Input: part model. Units: mm. Frame: model coordinates. Round coordinates to 2 decimals unless told otherwise and drop trailing zeros. Write each loop counter-clockwise with the first axis right and the second up, starting at its lowest first coordinate (ties: lowest second). Pieces come first, ordered by that corner, then holes. Notation, with made-up numbers: (65, 24) -> (78, 24) arc R25 ccw to (78, 57) -> close; hole circle Ø7 at (-12.75, 32). An arc over 180 degrees is marked (long way). Write item = value, one per line. Start each with the question number.
```python
from build123d import *

# Parameters (mm, degrees)
BOSS_EXTRUDE1_DEPTH  = 3.000000492
CUT_EXTRUDE1_DEPTH   = 4.000000492
BOSS_EXTRUDE3_DEPTH  = 4.999998957
SKETCH14_R           = 2.583283714
CUT_EXTRUDE6_DEPTH   = 8
M3_CLEARANCE_HOLE2_D = 3.2
M3_CLEARANCE_HOLE3_D = 3.2


with BuildPart() as part:
    # Sketch1 → Boss-Extrude1 (new body)
    with BuildSketch(Plane(origin=(0, 13.000000268, 0), x_dir=(1, 0, 0), z_dir=(0, 1, 0))):
        Polygon((0, -45.000001788), (76.499998569, -45.000001788), (76.499998569, -19.000001252), (53.249999881, 0), (23.250000551, 0), (0, -19.000001252), align=None)
    extrude(amount=-BOSS_EXTRUDE1_DEPTH)

    # Sketch2 → Cut-Extrude1 (cut, through all)
    with BuildSketch(Plane.XZ.offset(-9.999999776)):
        Polygon((24.331569672, 35.374999046), (24.056620896, 35.767666996), (23.717667907, 36.106623709), (23.324999958, 36.381572485), (22.890556604, 36.584153771), (22.427532822, 36.70822084), (21.949999034, 36.74999997), (21.472468972, 36.70822084), (21.00944519, 36.584153771), (20.574999973, 36.381572485), (20.182333887, 36.106623709), (19.843377173, 35.767666996), (19.56843026, 35.374999046), (19.365845248, 34.940555692), (19.241780043, 34.47753191), (19.200000912, 34.000001848), (19.241780043, 33.52246806), (19.365845248, 33.059444278), (19.56843026, 32.625000924), (19.843377173, 32.2323367), (20.182333887, 31.893379986), (20.574999973, 31.618431211), (21.00944519, 31.415846199), (21.472468972, 31.291779131), (21.949999034, 31.25), (22.427532822, 31.291779131), (22.890556604, 31.415846199), (23.324999958, 31.618431211), (23.717667907, 31.893379986), (24.056620896, 32.2323367), (24.331569672, 32.625000924), (24.534154683, 33.059444278), (24.658221751, 33.52246806), (24.700000882, 34.000001848), (24.658221751, 34.47753191), (24.534154683, 34.940555692), align=None)
    extrude(amount=-CUT_EXTRUDE1_DEPTH, mode=Mode.SUBTRACT)

    # Sketch4 → Boss-Extrude3 (add)
    with BuildSketch(Plane(origin=(0, 13.000000268, 0), x_dir=(-1, 0, 0), z_dir=(0, 1, 0))):
        Polygon((-41.949994862, 10.347297415), (-41.919611394, 9.999999776), (-41.949994862, 9.652704), (-42.040225118, 9.315960109), (-42.18756035, 9.000001475), (-42.387522757, 8.714426309), (-42.634036392, 8.467912674), (-42.919609696, 8.267950267), (-43.235570192, 8.120615035), (-43.572314084, 8.030384779), (-43.919611722, 8.000001311), (-44.266905636, 8.030384779), (-44.603649527, 8.120615035), (-44.919610023, 8.267950267), (-45.205187052, 8.467912674), (-45.451700687, 8.714426309), (-45.651663095, 9.000001475), (-45.798994601, 9.315960109), (-45.889224857, 9.652704), (-45.91961205, 9.999999776), (-45.889224857, 10.347297415), (-45.798994601, 10.684041306), (-45.651663095, 10.99999994), (-45.451700687, 11.285575107), (-45.205187052, 11.532089673), (-44.919610023, 11.732051149), (-44.603649527, 11.87938638), (-44.266905636, 11.969616637), (-43.919611722, 12.000001036), (-43.572314084, 11.969616637), (-43.235570192, 11.87938638), (-42.919609696, 11.732051149), (-42.634036392, 11.532089673), (-42.387522757, 11.285575107), (-42.18756035, 10.99999994), (-42.040225118, 10.684041306), align=None)
    extrude(amount=BOSS_EXTRUDE3_DEPTH)

    # Sketch14 → Cut-Extrude6 (cut)
    with BuildSketch(Plane(origin=(0, 13.000000268, 0), x_dir=(1, 0, 0), z_dir=(0, 1, 0))):
        with Locations((43.972754788, -10.139500391)):
            Circle(SKETCH14_R)
    extrude(amount=CUT_EXTRUDE6_DEPTH, mode=Mode.SUBTRACT)

    # M3 Clearance Hole2 (through all)
    with Locations(Plane(origin=(0, 13.000000268, 0), x_dir=(1, 0, 0), z_dir=(0, 1, 0))):
        with Locations((30.040436258, -10.00628369), (46.656531008, -10.00628369)):
            Hole(M3_CLEARANCE_HOLE2_D / 2)

    # M3 Clearance Hole3 (through all)
    with Locations(Plane(origin=(0, 13.000000268, 0), x_dir=(1, 0, 0), z_dir=(0, 1, 0))):
        with Locations((51.953516863, -32.727697483)):
            Hole(M3_CLEARANCE_HOLE3_D / 2)


solid = part.part
```
1. Section A-A (x = 51.5). Output: boundary loops of the cut face in (y, z), then the cut area to 3 significant figures.
2. Mould query, pull axis X, two halves, no side actions, for faces 1 (the cylindrical face through (28.514, 11.479, 9.526)), 2 (the flat face through (38, 12, 45)), 3 (the flat face through (76.5, 12, 32)). Classes: pulls with the +X half, pulls with the -X half, needs draft (parallel to the pull), parting line crosses it, or undercut.
3. Section D-D (x = 61). Output: boundary loops of the cut face in (y, z).
4. Pin query (flat end, axial travel): P1, Ø5, axis at x = 46.66, z = 10.01, coming from the -Y side; P2, Ø1.9, axis at x = 30.04, z = 10.01, coming from the +Y side. Return the tip coordinate at first contact, or that it passes through.
5. Section C-C (z = 13.5). Output: boundary loops of the cut face in (x, y), then the cut area to 3 significant figures.
6. Section B-B (y = 11.85). State how many separate pieces and enclosed holes the cut face has, then the cut area to 3 significant figures.
7. Line query: line 1 along X through (y, z) = (10.7, 10.5); line 2 along X through (y, z) = (11.3, 36); line 3 along Z through (x, y) = (22.5, 12.4). Output: solid intervals per line, ascending.
Check sheet entries:
q1.outline = (10, 0) -> (13, 0) -> (13, 31.19) -> (10, 31.19) -> close; (10, 34.26) -> (13, 34.26) -> (13, 45) -> (10, 45) -> close
q1.area = 126 mm2
q2.face_1 = undercut
q2.face_2 = needs draft
q2.face_3 = pulls with the +X half
q3.outline = (10, 6.33) -> (13, 6.33) -> (13, 45) -> (10, 45) -> close
q4.P1 = 10
q4.P2 = through
q5.outline = (6.73, 10) -> (69.77, 10) -> (69.77, 13) -> (6.73, 13) -> close
q5.area = 189 mm2
q6.separate_pieces = 1
q6.enclosed_holes = 4
q6.area = 2,950 mm2
q7.line_1 = 10.4 to 28.52, 31.56 to 45.13, 48.18 to 66.1
q7.line_2 = 0 to 20.08, 23.82 to 76.5
q7.line_3 = 0.61 to 31.31, 36.69 to 45
